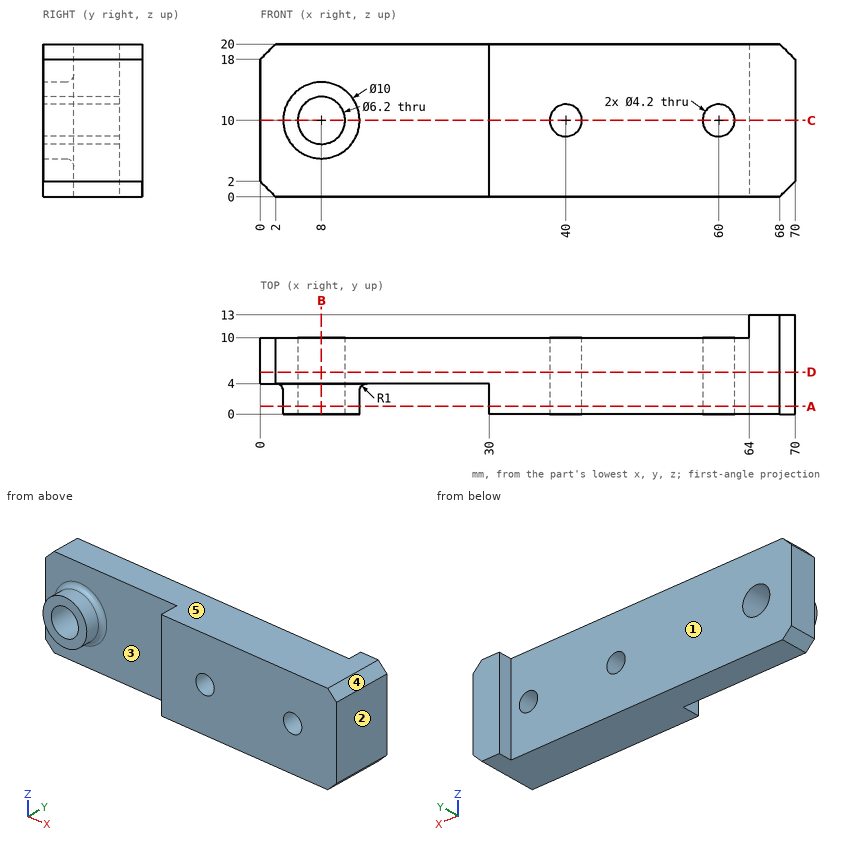
Geometry: see drawing. Coordinates: mm, zero at the bounding-box minimum. A direction names the side the tool comes from. Coordinates: 2 decimals unless noted, no trailing zeros. Order: outer loops, then holes, each group sorted by start corner. A loop starts at its lowest first (then second) coordinate and runs counter-clockwise, first axis right, second up. Notation, with made-up numbers: (-9.5, 27.25) - (-0.5, 27.25) arc R32 ccw to (-0.5, 61.25) - close; hole circle Ø11 at (44.25, 66). An arc over 180 degrees is marked (long way). Return JSON: item names as keys, results as strings.
Q1. Access query for the marked faces 1 and 2. Directions: +Z, -Z, +X, -X, +Y, -Y. A direction counts if a zero-diameter tool reaches every point of the face in a straight line with its end or side. Return the directions, or none.
The answers:
{"face 1": "+Z, -Z, -X, +Y", "face 2": "+Z, -Z, +X, +Y, -Y"}
Q2. Cut plane B-B (x = 8). Return loops of the section in (y, z).
The answers:
{"outline": "(0, 5) - (3, 5) arc R1 cw to (4, 4) - (4, 0) - (10, 0) - (10, 6.9) - (0, 6.9) - close; (0, 13.1) - (10, 13.1) - (10, 20) - (4, 20) - (4, 16) arc R1 cw to (3, 15) - (0, 15) - close"}
Q3. Draft query along X for the marked faces 3, 4 and 5. Return one class per face: +X half, -X half, draft (parallel to the pull), parting line (faces both ways), or undercut.
The answers:
{"face 3": "undercut", "face 4": "+X half", "face 5": "draft"}
Q4. Cut plane D-D (y = 5.5). Return loops of the section in (x, z), then the cut area to 3 significant figures.
The answers:
{"outline": "(0, 2) - (2, 0) - (68, 0) - (70, 2) - (70, 18) - (68, 20) - (2, 20) - (0, 18) - close; hole circle Ø6.2 at (8, 10); hole circle Ø4.2 at (40, 10); hole circle Ø4.2 at (60, 10)", "area": "1,330 mm2"}
Q5. Ray query, probe 1 along X at (y, z) = (2, 12.25); probe 2 along Z at (x, y) = (60, 6.5); probe 3 along Z at (x, y) = (8, 4.5). Return the intervals inside material, ascending.
The answers:
{"probe 1": "x = 3.53 to 5.87, 10.13 to 12.47, 30 to 70", "probe 2": "z = 0 to 7.9, 12.1 to 20", "probe 3": "z = 0 to 6.9, 13.1 to 20"}
Q6. Cut plane A-A (y = 1). Return loops of the section in (x, z).
The answers:
{"outline": "circle Ø10 at (8, 10); (30, 0) - (68, 0) - (70, 2) - (70, 18) - (68, 20) - (30, 20) - close; hole circle Ø6.2 at (8, 10); hole circle Ø4.2 at (40, 10); hole circle Ø4.2 at (60, 10)"}
Q7. First-contact query: pin 1 (4 mm diameter, centred on x = 56.5, z = 3, fed in from +Y); pin 2 (1.2 mm diameter, centred on y = 2, z = 12, fed in from -X); pin 3 (0.9 mm diameter, centred on y = 11, z = 5.5, fed in from -X). Flat tips, straight axial feed; report the tip coordinate or a pass-through.
The answers:
{"pin 1": "stops at y = 10", "pin 2": "stops at x = 3.2", "pin 3": "stops at x = 64"}
Q8. Cut plane C-C (z = 10). Return loops of the section in (x, y).
The answers:
{"outline": "(0, 4) - (2, 4) arc R1 cw to (3, 3) - (3, 0) - (4.9, 0) - (4.9, 10) - (0, 10) - close; (11.1, 0) - (13, 0) - (13, 3) arc R1 cw to (14, 4) - (30, 4) - (30, 0) - (37.9, 0) - (37.9, 10) - (11.1, 10) - close; (42.1, 0) - (57.9, 0) - (57.9, 10) - (42.1, 10) - close; (62.1, 0) - (70, 0) - (70, 13) - (64, 13) - (64, 10) - (62.1, 10) - close"}
